from build123d import *

# Parameters (mm, degrees)
F0_R     = 193.1582177029
F0_R_2   = 191.8011573182
F0_R_3   = 130.4635260733
F1_DEPTH = 74.2441564798
F5_R     = 5


# Not quite as in the source:
# - the program builds the solid bodies; features that only make, move or delete a surface that nothing else refers to are left out


with BuildPart() as f1:
    # F0 (on Top) → F1 (new body)
    with BuildSketch(Plane.XY):
        Circle(F0_R)
        Circle(F0_R_2, mode=Mode.SUBTRACT)
        Circle(F0_R_2)
        Circle(F0_R_3, mode=Mode.SUBTRACT)
    extrude(amount=F1_DEPTH)

    # F5
    f5_edges = [f1.edges().sort_by_distance(p)[0] for p in [
        (-193.158218, 0, 74.244156),
        (-130.463526, 0, 0),
        (-193.158218, 0, 0),
        (-130.463526, 0, 74.244156),
    ]]
    fillet(f5_edges, radius=F5_R)


solid = f1.part
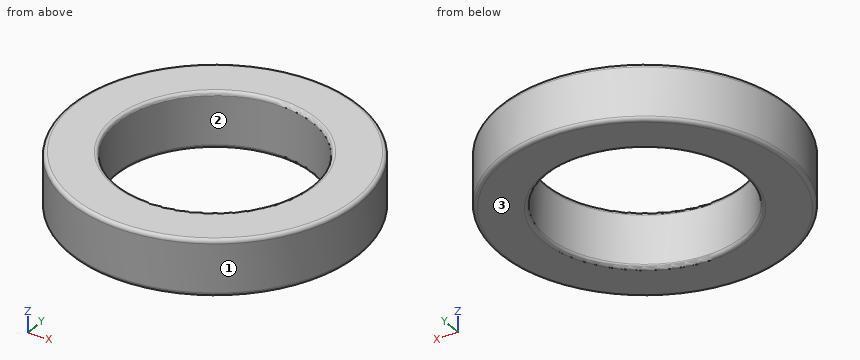
The listing builds one solid part. Answer for the finished solid, in the listing's coordinates (mm). Face numbers are marked on the shaded views. Round coordinates to 2 decimals unless told otherwise and drop trailing zeros. Loops run counter-clockwise (first coordinate to the right, second up) from the corner with the lowest first, then second, coordinate; pieces in that order, holes last. Notation, with made-up numbers: M 24,80 L 51,80 A12 cw 51,98 Z; hole C -1,-21.5 d8. An arc over 180 degrees is marked long. Return JSON: item names as keys, results as strings.
Q1. Each of these flat-tipped pins is pushed along its axis until it touches: pin 1 Ø12 at (x, z) = (41, 25) entering from +Y; pin 2 Ø8 at (x, z) = (-86.5, 37.5) entering from +Y; pin 3 Ø6 at (x, y) = (-140.5, 132.5) entering from -Z. Where does it stop, or does it pass through?
Results list:
{"pin 1": "stops at y = 189.96", "pin 2": "stops at y = 174.65", "pin 3": "stops at z = 0.4"}
Q2. Find the intervals of material crossed by line 1 along Y through (x, z) = (4, 14); line 2 along X through (y, z) = (1.5, 16.5); line 3 along Y through (x, z) = (-38, 56), in increasing order. Write a range as from..to.
Results list:
{"line 1": "y = -193.12..-130.4, 130.4..193.12", "line 2": "x = -193.15..-130.45, 130.45..193.15", "line 3": "y = -189.38..-124.81, 124.81..189.38"}
Q3. Find section A-A, the plane y = 0. Determine the outline of the cut face in (x, z).
Results list:
{"outline": "M -193.16,5 A5 ccw -188.16,0 L -135.46,0 A5 ccw -130.46,5 L -130.46,69.24 A5 ccw -135.46,74.24 L -188.16,74.24 A5 ccw -193.16,69.24 Z; M 130.46,5 A5 ccw 135.46,0 L 188.16,0 A5 ccw 193.16,5 L 193.16,69.24 A5 ccw 188.16,74.24 L 135.46,74.24 A5 ccw 130.46,69.24 Z"}
Q4. The mould has two halves that part along X. Classify the marked faces 1, 2 and 3: released by +X, released by -X, zero draft, split by the parting line, or undercut.
Results list:
{"face 1": "split by the parting line", "face 2": "undercut", "face 3": "zero draft"}
Q5. Find section C-C, the plane z = 54.5. Determine the outline of the cut face in (x, y).
Results list:
{"outline": "C 0,0 d386.32; hole C 0,0 d260.93"}
